The drawing under review shows one solid part. Ordinate dimensions are in mm from its lowest x, y, z. A direction names the side the tool comes from. Round coordinates to 2 decimals unless told otherwise and drop trailing zeros. Order: outer loops, then holes, each group sorted by start corner. A loop starts at its lowest first (then second) coordinate and runs counter-clockwise, first axis right, second up. Notation, with made-up numbers: (60, 79) -> (97, 79) arc R10 cw to (97, 93) -> close; hole circle Ø3 at (37, 75.5). An arc over 180 degrees is marked (long way). Use a Markdown table: item, result. Add a question column.
1) Wall thickness on line 1 along X through (y, z) = (4.5, 0.75); line 2 along Y through (x, z) = (30.7, 0.9); line 3 along Y through (x, z) = (30, 6.25): over which ranges is each line inside the solid? List them lowest first. Write a range as [from, to].
2) Machinability: for the marked faces 1, 2 and 3, which of the approach directions +Z, -Z, +X, -X, +Y, -Y give a long, thin tool a straight path to every point of the face, cutting with its end or side? Answer none if there is none.
3) Consider section D-D (z = 7.25). State the section outline as (x, y) points.
4) Consider section C-C (y = 47). State the section outline as (x, z) points.
5) Consider section B-B (x = 30.7). State the section outline as (y, z) points, plus the area to 3 significant figures.
6) Consider section A-A (y = 4.5). State the section outline as (x, z) points, plus the area to 3 significant figures.
7) Clearance check with flat-ended pins moving along their axes: P1, Ø3, axis at x = 9.5, y = 6.5, coming from the +Z side; P2, Ø1.8, axis at x = 6.8, y = 50.5, coming from the +Z side; P3, Ø5, axis at x = 15.5, y = 32, coming from the -Z side; P4, Ø6, axis at x = 17, z = 9.5, coming from the -Y side. State where each tip first meets the part, or that it passes through.
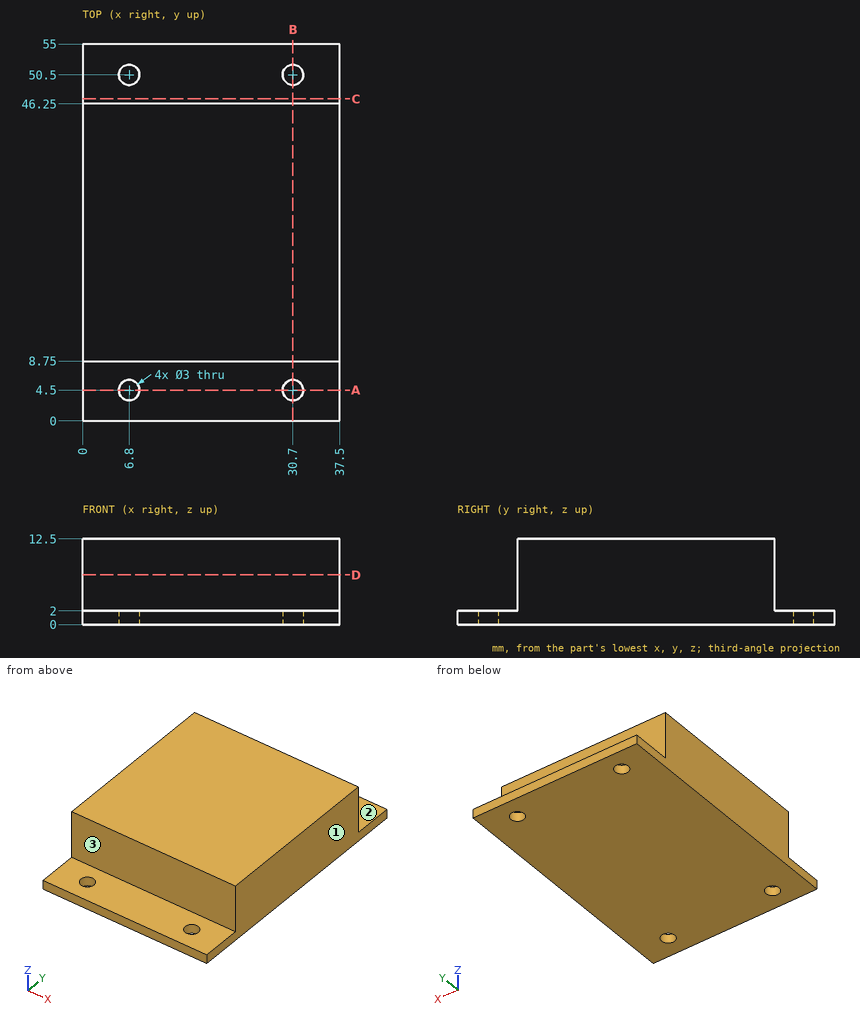
Results list:
| question | item | result |
|---|---|---|
| 1 | line 1 | [0, 5.3], [8.3, 29.2], [32.2, 37.5] |
| 1 | line 2 | [0, 3], [6, 49], [52, 55] |
| 1 | line 3 | [8.75, 46.25] |
| 2 | face 1 | +Z, -Z, +X, +Y, -Y |
| 2 | face 2 | +Z, +X, -X, +Y |
| 2 | face 3 | +Z, +X, -X, -Y |
| 3 | outline | (0, 8.75) -> (37.5, 8.75) -> (37.5, 46.25) -> (0, 46.25) -> close |
| 4 | outline | (0, 0) -> (37.5, 0) -> (37.5, 2) -> (0, 2) -> close |
| 5 | outline | (0, 0) -> (3, 0) -> (3, 2) -> (0, 2) -> close; (6, 0) -> (49, 0) -> (49, 2) -> (46.25, 2) -> (46.25, 12.5) -> (8.75, 12.5) -> (8.75, 2) -> (6, 2) -> close; (52, 0) -> (55, 0) -> (55, 2) -> (52, 2) -> close |
| 5 | area | 492 mm2 |
| 6 | outline | (0, 0) -> (5.3, 0) -> (5.3, 2) -> (0, 2) -> close; (8.3, 0) -> (29.2, 0) -> (29.2, 2) -> (8.3, 2) -> close; (32.2, 0) -> (37.5, 0) -> (37.5, 2) -> (32.2, 2) -> close |
| 6 | area | 63.0 mm2 |
| 7 | P1 | z = 2 |
| 7 | P2 | through |
| 7 | P3 | z = 0 |
| 7 | P4 | y = 8.75 |
